Build history of the part. All positions in model axes, mm. A direction names the side the tool comes from. Coordinates: 2 decimals unless noted, no trailing zeros. Order: outer loops, then holes, each group sorted by start corner. A loop starts at its lowest first (then second) coordinate and runs counter-clockwise, first axis right, second up. Notation, with made-up numbers: M 50.5,45 L 82.5,45 A24 ccw 82.5,57 Z; hole C 36.25,-4 d2. An arc over 180 degrees is marked long. Write item = value, one per line. Start each with the question number.
Q1. Band-saw the part on C-C on x = -7.5. Write the cut outline in (y, z), plus the area to 3 significant figures.
Q2. Band-saw the part on B-B on y = -5.5. Write the cut outline in (x, z), plus the area to 3 significant figures.
Q3. Pull direction Z, two halves, no side cores. Call faces 1 (the face through (-1, 0, 0)), 2 (the face through (-17.859, 10.797, 106.521)), 3 (the face through (-0.716, -19.014, 58.402)): released by +Z, released by -Z, zero draft, split by the parting line, or undercut.
Q4. Drill centre lines: probe 1 along X at (y, z) = (8, 39.5); probe 2 along Z at (x, y) = (4, -1); probe 3 along Y at (x, z) = (-19, 36). Where is each one in solid material? Low to high.
Q5. Pin check, flat tips, straight feed: P1, Ø1, axis at x = -26, z = 54.5, coming from the -Y side; P2, Ø3, axis at y = 3, z = 74, coming from the -X side; P3, Ø8, axis at x = -14, z = 95.5, coming from the +Y side. Stop position of each tip, or through.
Q6. Band-saw the part on A-A on z = 36. Write the cut outline in (x, y), plus the area to 3 significant figures.
Q7. Band-saw the part on D-D on z = 51. Write the cut outline in (x, y), plus the area to 3 significant figures.
Q8. 3-axis set-ups, long thin cutter, end or side, ignore diameter. For faces 4 (the face through (17.797, 10.859, 106.521)), 5 (the face through (-34.768, 3.542, 92.783)), 6 (the face through (-2, -19, 71)), 7 (the face through (-2, 19, 71)), 8 (the face through (34.768, 3.542, 92.783)): which of +Z, -Z, +X, -X, +Y, -Y reach the whole face in a straight line?
```python
from build123d import *

# Parameters (mm, degrees)
SKETCH_1_W          = 72
SKETCH_1_H          = 40
EXTRUDE_1_DEPTH     = 108
SKETCH_1_2_W        = 72
SKETCH_1_2_H        = 40
EXTRUDE_2_DEPTH     = 105
CUT_EXTRUDE_1_DEPTH = 2.5
CUT_EXTRUDE_2_DEPTH = 2
CUT_EXTRUDE_3_DEPTH = 3


with BuildPart() as part:
    # 草图1 → 凸台-拉伸1 (new body)
    with BuildSketch(Plane.XY):
        Rectangle(SKETCH_1_W, SKETCH_1_H)
    extrude(amount=EXTRUDE_1_DEPTH)

    # 草图1<2> → 凸台-拉伸2 (add)
    with BuildSketch(Plane.XY):
        Rectangle(SKETCH_1_2_W, SKETCH_1_2_H)
    extrude(amount=EXTRUDE_2_DEPTH)

    # 草图2 → 切除-拉伸1 (cut)
    with BuildSketch(Plane.ZY.offset(36)):
        with BuildLine():
            Line((26, 12), (88, 12))
            ThreePointArc((88, 12), (91.170727435, 10.300174957), (92.572660223, 6.986943589))
            Line((92.572660223, 6.986943589), (93, 0))
            Line((93, 0), (92.572660223, -6.986943589))
            ThreePointArc((92.572660223, -6.986943589), (91.170727435, -10.300174957), (88, -12))
            Line((88, -12), (26, -12))
            ThreePointArc((26, -12), (22.829272565, -10.300174957), (21.427339777, -6.986943589))
            Line((21.427339777, -6.986943589), (21, 0))
            Line((21, 0), (21.427339777, 6.986943589))
            ThreePointArc((21.427339777, 6.986943589), (22.829272565, 10.300174957), (26, 12))
        make_face()
    cut_extrude_1 = extrude(amount=-CUT_EXTRUDE_1_DEPTH, mode=Mode.SUBTRACT)

    # 草图3 → 切除-拉伸2 (cut)
    with BuildSketch(Plane(origin=(0, 20, 0), x_dir=(1, 0, 0), z_dir=(0, 1, 0))):
        with BuildLine():
            Line((25, -100), (-24.964466094, -100))
            ThreePointArc((-24.964466094, -100), (-27.274164925, -98.456708581), (-26.732233047, -95.732233047))
            Line((-26.732233047, -95.732233047), (23.732233047, -45.267766953))
            ThreePointArc((23.732233047, -45.267766953), (26.456708581, -44.725835075), (28, -47.035533906))
            Line((28, -47.035533906), (28, -97))
            ThreePointArc((28, -97), (27.121320344, -99.121320344), (25, -100))
        make_face()
        with BuildLine():
            Line((-31, -85.064971157), (-31, -22.686291501))
            ThreePointArc((-31, -22.686291501), (-29.828427125, -19.857864376), (-27, -18.686291501))
            Line((-27, -18.686291501), (25, -18.686291501))
            ThreePointArc((25, -18.686291501), (27.121320344, -19.564971157), (28, -21.686291501))
            Line((28, -21.686291501), (28, -27.201010127))
            ThreePointArc((28, -27.201010127), (27.543277195, -29.497110721), (26.242640687, -31.443650814))
            Line((26.242640687, -31.443650814), (-28.439339828, -86.125631329))
            ThreePointArc((-28.439339828, -86.125631329), (-30.074025149, -86.450790456), (-31, -85.064971157))
        make_face()
    cut_extrude_2 = extrude(amount=-CUT_EXTRUDE_2_DEPTH, mode=Mode.SUBTRACT)

    # 镜向1: 切除-拉伸2 across plane
    add(cut_extrude_2.mirror(Plane.ZX), mode=Mode.SUBTRACT)

    # 镜向2: 切除-拉伸1 across plane
    add(cut_extrude_1.mirror(Plane.ZY), mode=Mode.SUBTRACT)

    # 草图5 → 切除-拉伸3 (cut)
    with BuildSketch(Plane.XY.offset(108)):
        with BuildLine():
            Line((15, -12), (-15, -12))
            ThreePointArc((-15, -12), (-17.828427125, -10.828427125), (-19, -8))
            Line((-19, -8), (-19, 8))
            ThreePointArc((-19, 8), (-17.828427125, 10.828427125), (-15, 12))
            Line((-15, 12), (15, 12))
            ThreePointArc((15, 12), (17.828427125, 10.828427125), (19, 8))
            Line((19, 8), (19, -8))
            ThreePointArc((19, -8), (17.828427125, -10.828427125), (15, -12))
        make_face()
    extrude(amount=-CUT_EXTRUDE_3_DEPTH, mode=Mode.SUBTRACT)


solid = part.part
```
Recorded:
q1.outline = M -20,0 L 20,0 L 20,18.69 L 18,18.69 L 18,65.19 L 20,65.19 L 20,76.5 L 18,76.5 L 18,100 L 20,100 L 20,108 L 12,108 L 12,105 L -12,105 L -12,108 L -20,108 L -20,100 L -18,100 L -18,76.5 L -20,76.5 L -20,65.19 L -18,65.19 L -18,18.69 L -20,18.69 Z
q1.area = 3,970 mm2
q2.outline = M -36,0 L 36,0 L 36,21.34 L 33.5,21.34 L 33.5,92.66 L 36,92.66 L 36,108 L 19,108 L 19,105 L -19,105 L -19,108 L -36,108 L -36,92.66 L -33.5,92.66 L -33.5,21.34 L -36,21.34 Z
q2.area = 7,310 mm2
q3.face_1 = released by -Z
q3.face_2 = zero draft
q3.face_3 = undercut
q4.probe_1 = -33.5 to 33.5
q4.probe_2 = 0 to 105
q4.probe_3 = -18 to 18
q5.P1 = -18
q5.P2 = -33.5
q5.P3 = 18
q6.outline = M -36,-20 L -31,-20 L -31,-18 L 21.69,-18 L 21.69,-20 L 36,-20 L 36,-12 L 33.5,-12 L 33.5,12 L 36,12 L 36,20 L 21.69,20 L 21.69,18 L -31,18 L -31,20 L -36,20 L -36,12 L -33.5,12 L -33.5,-12 L -36,-12 Z
q6.area = 2,550 mm2
q7.outline = M -36,-20 L -31,-20 L -31,-18 L 6.69,-18 L 6.69,-20 L 18,-20 L 18,-18 L 28,-18 L 28,-20 L 36,-20 L 36,-12 L 33.5,-12 L 33.5,12 L 36,12 L 36,20 L 28,20 L 28,18 L 18,18 L 18,20 L 6.69,20 L 6.69,18 L -31,18 L -31,20 L -36,20 L -36,12 L -33.5,12 L -33.5,-12 L -36,-12 Z
q7.area = 2,570 mm2
q8.face_4 = +Z
q8.face_5 = -X
q8.face_6 = -Y
q8.face_7 = +Y
q8.face_8 = +X
